For this review, take the finished solid that the model builds, in its own axes (mm). Coordinates: 2 decimals unless noted, no trailing zeros. Write each loop counter-clockwise with the first axis right and the second up, starting at its lowest first coordinate (ties: lowest second). Pieces come first, ordered by that corner, then holes. Notation, with made-up numbers: (81.25, 35.5) -> (109.25, 35.5) arc R16 cw to (109.25, 51.5) -> close; hole circle Ø4 at (17.5, 30). An arc over 180 degrees is marked (long way). Put each result on its own line as item: value. Start each with the question number.
Item 1: Consider section A-A on z = -3.5. Give the boundary of the cut face in (x, y).
Item 2: Consider section D-D on z = -12. Give the boundary of the cut face in (x, y), and give its area (3 significant figures).
Item 3: The part is to be moulded in two halves that separate along X. For faces 1 (the flat face through (0, -31, 0)), 2 (the flat face through (10, -31, 0)), 3 (the flat face through (5, -30, -15.451)), say which applies: +X half, -X half, draft (parallel to the pull), parting line (faces both ways), or undercut.
Item 4: Insertion check: P1, Ø3, axis at x = 1.5, z = -7, coming from the +Y side; P2, Ø8.5, axis at y = -104.45, z = -0.45, coming from the +X side; P3, Ø2, axis at x = 1.5, z = -11.5, coming from the +Y side. Each pin has a flat end and moves straight along its axis. Give the tip position at first contact, or say it passes through.
Item 5: Consider section B-B on x = 8.25. Give the boundary of the cut face in (y, z).
Item 6: To check wall thickness, follow L1, parallel to Y at x = 7.25, z = 0; L2, parallel to Z at x = 3, y = -104; L3, parallel to Y at x = 6, z = -4. State the ranges of each line that lie inside material, in increasing order.
Item 7: Consider section C-C on z = 7.75. Give the boundary of the cut face in (x, y), and give its area (3 significant figures).
Solid Edge part; units mm, degrees
sketch "Sketch1" plane through (0, 0, 0) normal (1, 0, 0) x (0, 1, 0)
  line L0 (-104.4456, 14.5486) -> (45.5544, 14.5486)
  arc A0 (45.5544, -15.4514) -> (45.5544, 14.5486) centre (45.5544, -0.4514) ccw
  line L1 (-104.4456, -15.4514) -> (45.5544, -15.4514)
  arc A1 (-104.4456, 14.5486) -> (-104.4456, -15.4514) centre (-104.4456, -0.4514) ccw
extrude "Protrusion1" add sketch "Sketch1" along normal blind 10
sketch "Sketch2" plane through (0, 0, 0) normal (1, 0, 0) x (0, 1, 0)
  circle A0 centre (-104.4456, -0.4514) radius 4.7659
  circle A1 centre (45.5544, -0.4514) radius 4.7659
extrude "Cutout1" cut sketch "Sketch2" along normal blind 53.975
Return value:
1. outline: (0, -119.13) -> (10, -119.13) -> (10, -108.11) -> (0, -108.11) -> close; (0, -100.78) -> (10, -100.78) -> (10, 41.89) -> (0, 41.89) -> close; (0, 49.22) -> (10, 49.22) -> (10, 60.24) -> (0, 60.24) -> close
2. outline: (0, -114.02) -> (10, -114.02) -> (10, 55.13) -> (0, 55.13) -> close
2. area: 1,690 mm^2
3. face 1: -X half
3. face 2: +X half
3. face 3: draft
4. P1: y = 59.68
4. P2: through
4. P3: y = 56.69
5. outline: (-104.45, -15.45) -> (45.55, -15.45) arc R15 ccw to (45.55, 14.55) -> (-104.45, 14.55) arc R15 ccw to start; hole circle Ø9.53 at (-104.45, -0.45); hole circle Ø9.53 at (45.55, -0.45)
6. L1: -119.44 to -109.19, -99.7 to 40.81, 50.3 to 60.55
6. L2: -15.45 to -5.2, 4.29 to 14.55
6. L3: -119.02 to -107.63, -101.26 to 42.37, 48.74 to 60.13
7. outline: (0, -117) -> (10, -117) -> (10, 58.11) -> (0, 58.11) -> close
7. area: 1,750 mm^2
